Autodesk Inventor part; units mm, degrees
ref_plane "YZ Plane" through (0, 0, 0) normal (1, 0, 0) x (0, 1, 0)
ref_plane "XZ Plane" through (0, 0, 0) normal (0, 1, 0) x (-1, 0, 0)
ref_plane "XY Plane" through (0, 0, 0) normal (0, 0, 1) x (1, 0, 0)
sketch "Sketch1" plane through (0, 0, 0) normal (0, 0, 1) x (1, 0, 0)
  circle A0 centre (0, 0) radius 5.3975
  dimension "d0" = 10.795
extrude "Extrusion1" add sketch "Sketch1" along normal blind 12.7
thread "Thread1"
sketch "Sketch2" plane through (0, 0, 12.7) normal (0, 0, 1) x (1, 0, 0)
  circle A0 centre (0, 0) radius 5.3975
  line L0 (0, 7.3323) -> (6.35, 3.6662)
  line L1 (6.35, 3.6662) -> (6.35, -3.6662)
  line L2 (6.35, -3.6662) -> (0, -7.3323)
  line L3 (0, -7.3323) -> (-6.35, -3.6662)
  line L4 (-6.35, -3.6662) -> (-6.35, 3.6662)
  line L5 (-6.35, 3.6662) -> (0, 7.3323)
  dimension "d5" = 12.7
  dimension "d6" = 0
extrude "Extrusion2" add sketch "Sketch2" along normal blind 6.35 contours A0 | L0 L1 L2 L3 L4 L5
sketch "Sketch3" plane through (0, 0, 19.05) normal (0, 0, 1) x (1, 0, 0)
  line L0 (0, 7.3323) -> (6.35, 3.6662)
  circle A0 centre (0, 0) radius 6.35
extrude "Extrusion3" add sketch "Sketch3" along normal blind 2.54
sketch "Sketch4" plane through (0, 0, 21.59) normal (0, 0, 1) x (1, 0, 0)
  circle A0 centre (0, 0) radius 6.35
  circle A1 centre (0, 0) radius 3.175
  dimension "d11" = 6.35
extrude "Extrusion4" cut sketch "Sketch4" against normal through all contours A1
properties part number "Pnewmatic Screw Part 1 1764"
CAD build for the part. Positions are in the model's coordinates, mm. A direction names the side the tool comes from. Give positions to 0.01 mm unless a question says otherwise; leave off trailing zeros. Order: outer loops, then holes, each group sorted by start corner. A loop starts at its lowest first (then second) coordinate and runs counter-clockwise, first axis right, second up. Notation, with made-up numbers: (13.25, -3) -> (50.25, -3) arc R23 ccw to (50.25, 17) -> close; hole circle Ø8 at (26.25, -17). An arc over 180 degrees is marked (long way). Return JSON: item names as keys, results as strings.
Q1. Mould opens along Y. For faces 4 (the face through (6, -3, 19.05)), 5 (the face through (-1.38, 6.2, 20.3)), 6 (the face through (-0.69, -3.1, 10.95)) say: pulls with the +Y half, pulls with the -Y half, needs draft (parallel to the pull), parting line crosses it, or undercut.
Working result:
{"face 4": "needs draft", "face 5": "parting line crosses it", "face 6": "undercut"}
Q2. Which spindle directions (+Z, -Z, +X, -X, +Y, -Y) get a long thin tool onto all of the face, cutting with end or side? Do faces 1 (the face through (-6, 3, 19.05)), 2 (the face through (6, 3, 19.05)), 3 (the face through (-3, -5, 12.7)). Say none if no direction does.
Working result:
{"face 1": "+Z, -X, +Y", "face 2": "+Z, +X, +Y", "face 3": "-Z"}
Q3. Drill centre lines: line 1 (Y direction, x = 0, z = 7.25) (1 decimal); line 2 (Z direction, x = 4.75, y = -3.25); line 3 (X direction, y = 0.75, z = 16). Where is each one in solid material? Low to high.
Working result:
{"line 1": "-5.4 to -3.2, 3.2 to 5.4", "line 2": "12.7 to 21.59", "line 3": "-6.35 to -3.09, 3.09 to 6.35"}
Q4. Flat gauge pins, fed straight in: pin 1 (6 mm diameter, centred on x = -2.5, z = 8, fed in from +Y); pin 2 (1.5 mm diameter, centred on x = -3, z = 16, fed in from +Y); pin 3 (5 mm diameter, centred on y = -2.5, z = 7.5, fed in from -X); pin 4 (5.5 mm diameter, centred on x = 0, y = 0, fed in from +Z). Where does each tip first touch, or does it go through?
Working result:
{"pin 1": "y = 5.4", "pin 2": "y = 6.03", "pin 3": "x = -5.4", "pin 4": "through"}
Q5. Saw through at D-D (y = -4.5). Write the cut outline in (x, z).
Working result:
{"outline": "(-4.91, 12.7) -> (-2.98, 12.7) -> (-2.98, 0) -> (2.98, 0) -> (2.98, 12.7) -> (4.91, 12.7) -> (4.91, 19.05) -> (4.48, 19.05) -> (4.48, 21.59) -> (-4.48, 21.59) -> (-4.48, 19.05) -> (-4.91, 19.05) -> close"}
Q6. Saw through at B-B (z = 19.75). Write the cut outline in (x, y) (3 decimals).
Working result:
{"outline": "circle Ø12.7 at (0, 0); hole circle Ø6.35 at (0, 0)"}
Q7. Saw through at A-A (x = -0.25). Write the cut outline in (y, z).
Working result:
{"outline": "(-7.19, 12.7) -> (-5.39, 12.7) -> (-5.39, 0) -> (-3.17, 0) -> (-3.17, 21.59) -> (-6.35, 21.59) -> (-6.35, 19.05) -> (-7.19, 19.05) -> close; (3.17, 0) -> (5.39, 0) -> (5.39, 12.7) -> (7.19, 12.7) -> (7.19, 19.05) -> (6.35, 19.05) -> (6.35, 21.59) -> (3.17, 21.59) -> close"}
